Source: CAD feature listing. Evaluate the final solid. Frame: model axes, mm. A direction names the side the tool comes from. Give positions to 0.01 mm unless a question says otherwise; leave off trailing zeros. Order: outer loops, then holes, each group sorted by start corner. A loop starts at its lowest first (then second) coordinate and runs counter-clockwise, first axis right, second up.
```python
from build123d import *

# Parameters (mm, degrees)
BOSS_EXTRUDE1_DEPTH = 5
SKETCH2_R           = 7.5
SKETCH2_R_2         = 3
BOSS_EXTRUDE2_DEPTH = 57.735026919
CUT_EXTRUDE1_DEPTH  = 57.735026919
CUT_EXTRUDE2_DEPTH  = 5
FILLET1_R           = 3
CUT_EXTRUDE3_DEPTH  = 0.5
CHAMFER1_SIZE       = 4
CHAMFER1_SIZE2      = 20
BOSS_EXTRUDE3_START = 3
SKETCH5_R           = 1.5
BOSS_EXTRUDE3_DEPTH = 3
FILLET2_R           = 1


with BuildPart() as part:
    # Sketch1 → Boss-Extrude1 (new body)
    with BuildSketch(Plane(origin=(0, 0, 0), x_dir=(1, 0, 0), z_dir=(0, 1, 0))):
        Polygon((-28.867513459, 50), (-28.867513459, 70), (28.867513459, 70), (28.867513459, 50), (0, 0), align=None)
    extrude(amount=BOSS_EXTRUDE1_DEPTH)

    # Sketch2 → Boss-Extrude2 (add)
    with BuildSketch(Plane(origin=(28.867513459, 0, 0), x_dir=(0, 0, -1), z_dir=(1, 0, 0))):
        with Locations((62.5, 2.5)):
            Circle(SKETCH2_R)
        with Locations((62.5, 2.5)):
            Circle(SKETCH2_R_2, mode=Mode.SUBTRACT)
    extrude(amount=-BOSS_EXTRUDE2_DEPTH)

    # Sketch2<2> → Cut-Extrude1 (cut)
    with BuildSketch(Plane(origin=(28.867513459, 0, 0), x_dir=(0, 0, -1), z_dir=(1, 0, 0))):
        with BuildLine():
            ThreePointArc((65.5, 2.5), (65.143382037, 3.918637165), (64.158312395, 5))
            Line((64.158312395, 5), (60.841687605, 5))
            ThreePointArc((60.841687605, 5), (59.5, 2.5), (60.841687605, 0))
            Line((60.841687605, 0), (64.158312395, 0))
            ThreePointArc((64.158312395, 0), (65.143382037, 1.081362835), (65.5, 2.5))
        make_face()
        with BuildLine():
            Line((60.841687605, 5), (64.158312395, 5))
            ThreePointArc((64.158312395, 5), (62.5, 5.5), (60.841687605, 5))
        make_face()
        with BuildLine():
            ThreePointArc((60.841687605, 0), (62.5, -0.5), (64.158312395, 0))
            Line((64.158312395, 0), (60.841687605, 0))
        make_face()
        with BuildLine():
            ThreePointArc((69.571067812, 5), (69.891989197, 3.76826484), (70, 2.5))
            Line((70, 2.5), (70, 5))
            Line((70, 5), (69.571067812, 5))
        make_face()
        with BuildLine():
            Line((70, 0), (70, 2.5))
            ThreePointArc((70, 2.5), (69.891989197, 1.23173516), (69.571067812, 0))
            Line((69.571067812, 0), (70, 0))
        make_face()
    extrude(amount=-CUT_EXTRUDE1_DEPTH, mode=Mode.SUBTRACT)

    # Sketch3 → Cut-Extrude2 (cut)
    with BuildSketch(Plane(origin=(0, 5, 0), x_dir=(1, 0, 0), z_dir=(0, 1, 0))):
        Polygon((-2.5, 4.330127019), (2.5, 4.330127019), (0, 0), align=None)
    extrude(amount=-CUT_EXTRUDE2_DEPTH, mode=Mode.SUBTRACT)

    # Fillet1
    fillet1_edges = [part.edges().sort_by_distance(p)[0] for p in [
        (0, 0, -55.428932188),
        (0, 5, -55.428932188),
    ]]
    fillet(fillet1_edges, radius=FILLET1_R)

    # Sketch4 → Cut-Extrude3 (cut)
    with BuildSketch(Plane(origin=(0, 0, 0), x_dir=(0.5000000000000001, 0, -0.8660254037844386), z_dir=(0.8660254037844386, 0, 0.5000000000000001))):
        with BuildLine():
            Line((57.735026919, 0), (60.814377774, 0))
            add(Edge.make_bspline(
                [(63.027511115, -1.428571429), (62.266746529, 0), (60.814377774, 0)],
                knots=[2.122113296, 2.122113296, 2.122113296, 3.141592654, 3.141592654, 3.141592654], degree=2, weights=[1, 0.872871561, 1]))
            add(Edge.make_bspline(
                [(63.027511115, -1.428571429), (75.055534995, -24.014916241), (75.055534995, 2.5), (75.055534995, 29.014916241), (63.027511115, 6.428571429)],
                knots=[5.26370595, 5.26370595, 5.26370595, 7.853981634, 7.853981634, 10.444257318, 10.444257318, 10.444257318], degree=2, weights=[1, 0.27218062, 1, 0.27218062, 1]))
            add(Edge.make_bspline(
                [(60.814377774, 5), (62.266746529, 5), (63.027511115, 6.428571429)],
                knots=[3.141592654, 3.141592654, 3.141592654, 4.161072011, 4.161072011, 4.161072011], degree=2, weights=[1, 0.872871561, 1]))
            Line((60.814377774, 5), (57.735026919, 5))
            Line((57.735026919, 5), (5, 5))
            Line((5, 5), (2.5, 5))
            Line((2.5, 5), (2.5, 0))
            Line((2.5, 0), (5, 0))
            Line((5, 0), (57.735026919, 0))
        make_face()
    cut_extrude3 = extrude(amount=-CUT_EXTRUDE3_DEPTH, mode=Mode.SUBTRACT)

    # Mirror1: Cut-Extrude3 across plane
    add(cut_extrude3.mirror(Plane(origin=(0, 0, 0), x_dir=(0, 0, 1), z_dir=(1, 0, 0))), mode=Mode.SUBTRACT)

    # Chamfer1
    chamfer1_edges = [part.edges().sort_by_distance(p)[0] for p in [
        (0, 0, -4.330127019),
    ]]
    chamfer1_side = [part.faces().sort_by_distance(p)[0] for p in [
        (0, 2.5, -4.330127019),
    ]]
    chamfer(chamfer1_edges, length=CHAMFER1_SIZE, length2=CHAMFER1_SIZE2, reference=chamfer1_side[0])

    # Sketch5 → Boss-Extrude3 (add)
    with BuildSketch(Plane(origin=(0, 0, 0), x_dir=(0, 0, -1), z_dir=(1, 0, 0)).offset(BOSS_EXTRUDE3_START)):
        with BuildLine():
            Line((35.307692308, 10.538461538), (33, 5))
            Line((33, 5), (45, 5))
            Line((45, 5), (42.692307692, 10.538461538))
            ThreePointArc((42.692307692, 10.538461538), (39, 13), (35.307692308, 10.538461538))
        make_face()
        with Locations((39, 9)):
            Circle(SKETCH5_R, mode=Mode.SUBTRACT)
    boss_extrude3 = extrude(amount=BOSS_EXTRUDE3_DEPTH)

    # Mirror2: Boss-Extrude3 across plane
    add(boss_extrude3.mirror(Plane(origin=(0, 0, 0), x_dir=(0, 0, 1), z_dir=(1, 0, 0))))

    # Fillet2
    fillet2_edges = [part.edges().sort_by_distance(p)[0] for p in [
        (6, 5, -39),
        (3, 5, -39),
        (4.5, 5, -33),
        (4.5, 5, -45),
        (-6, 5, -39),
        (-4.5, 5, -45),
        (-4.5, 5, -33),
        (-3, 5, -39),
    ]]
    fillet(fillet2_edges, radius=FILLET2_R)


solid = part.part
```
1) Section query B-B, the plane x = 0. Return the cut outline in (y, z), and give its area (3 significant figures).
Report:
outline: (-1.43, -56.11) arc R7.5 ccw (long way) to (6.43, -56.11) arc R3 cw to (5, -53.56) - (5, -4.33) - (4, -4.33) - (0, -24.33) - (0, -53.56) arc R3 cw to start; hole circle Ø6 at (2.5, -62.5)
area: 364 mm2
2) Material intervals for L1, parallel to Y at x = 5.3, z = -39; L2, parallel to X at y = 12, z = -40; L3, parallel to Y at x = -25, z = -51.5, sorted ascending.
Report:
L1: y = 0 to 7.5, 10.5 to 13
L2: x = -6 to -3, 3 to 6
L3: y = 0 to 5
3) Pin query (flat end, axial travel): pin 1 (6 mm diameter, centred on x = 17, z = -40.5, fed in from -Y); pin 2 (8 mm diameter, centred on x = -21.5, z = -45.5, fed in from +Y); pin 3 (6 mm diameter, centred on x = -8.5, y = 9.5, fed in from -Z). Return the tip coordinate at first contact, or that it passes through.
Report:
pin 1: stops at y = 0
pin 2: stops at y = 5
pin 3: stops at z = -68.84
4) Section query A-A, the plane z = -39. Return the cut outline in (x, y), and give its area (3 significant figures).
Report:
outline: (-21.94, 0) - (21.94, 0) - (21.94, 5) - (7, 5) arc R1 cw to (6, 6) - (6, 7.5) - (3, 7.5) - (3, 6) arc R1 cw to (2, 5) - (-2, 5) arc R1 cw to (-3, 6) - (-3, 7.5) - (-6, 7.5) - (-6, 6) arc R1 cw to (-7, 5) - (-21.94, 5) - close; (-6, 10.5) - (-3, 10.5) - (-3, 13) - (-6, 13) - close; (3, 10.5) - (6, 10.5) - (6, 13) - (3, 13) - close
area: 250 mm2
5) Section query D-D, the plane x = -9.5. Return the cut outline in (y, z), and give its area (3 significant figures).
Report:
outline: (-1.43, -56.11) arc R7.5 ccw (long way) to (6.43, -56.11) arc R3 cw to (5, -53.56) - (5, -17.45) - (1.38, -17.45) - (0, -24.33) - (0, -53.56) arc R3 cw to start; hole circle Ø6 at (2.5, -62.5)
area: 333 mm2
6) Draft query along Z for faces 6 (the cylindrical face through (4, 13, -39)), 7 (the cylindrical face through (4.5, 8.1, -37.8)), 8 (the flat face through (-28.868, 2, -58)). Return one class per face: +Z half, -Z half, draft (parallel to the pull), parting line (faces both ways), or undercut.
Report:
face 6: parting line
face 7: undercut
face 8: draft
7) Reachability of faces 1 (the flat face through (0, 0, -42)), 2 (the flat face through (-6, 7.99, -37.68)), 3 (the flat face through (6, 7.99, -37.68)), 4 (the flat face through (-4.478, 8.042, -43.732)), 5 (the flat face through (-3, 7.99, -37.68)) from +Z, -Z, +X, -X, +Y, -Y: full face, straight path, thin tool, end or side. Return the list, or none.
Report:
face 1: +Z, +X, -X, -Y
face 2: +Z, -X, +Y
face 3: +Z, +X, +Y
face 4: +X, -X, +Y
face 5: +Z, +Y
8) Section query C-C, the plane y = 9. Return the cut outline in (x, z), and give its area (3 significant figures).
Report:
outline: (-28.87, -66.24) - (28.87, -66.24) - (28.87, -58.76) - (-28.87, -58.76) - close; (-6, -43.33) - (-3, -43.33) - (-3, -40.5) - (-6, -40.5) - close; (-6, -37.5) - (-3, -37.5) - (-3, -34.67) - (-6, -34.67) - close; (3, -43.33) - (6, -43.33) - (6, -40.5) - (3, -40.5) - close; (3, -37.5) - (6, -37.5) - (6, -34.67) - (3, -34.67) - close
area: 466 mm2
